The listing builds one solid part. Answer for the finished solid, in the listing's coordinates (mm). Give positions to 0.01 mm unless a question says otherwise; leave off trailing zeros. Write each loop counter-clockwise with the first axis right and the second up, starting at its lowest first coordinate (ties: lowest second). Pieces come first, ordered by that corner, then holes. Notation, with made-up numbers: (54, 23) - (103, 23) arc R26 cw to (103, 50) - close; hole circle Ø6 at (57.25, -10). An arc over 180 degrees is marked (long way). Answer as CSV lines item,"result". Start each with the question number.
(1) Find section A-A (x = 1). Write down the section's boundary in (y, z) (3 decimals).
(2) Find section C-C (x = 4.75). Write down the section's boundary in (y, z) (3 decimals), then the cut area to 3 significant figures.
(3) Each of these flat-tipped pins is pushed along its axis until it touches: pin 1 Ø1.2 at (x, z) = (9, 28.5) entering from -Y; pin 2 Ø0.7 at (y, z) = (7.5, 43.5) entering from -X; pin 3 Ø1.6 at (x, z) = (7.5, 28.5) entering from -Y. Where does it stop, or does it pass through?
(4) Find section B-B (y = 0.75). Write down the section's boundary in (x, z) (3 decimals), then the cut area to 3 significant figures.
(5) Straight lines are drawn through the part: probe 1 along X at (y, z) = (-5.25, 23.5) (3 decimals); probe 2 along X at (y, z) = (2.5, 11.5) (3 decimals); probe 3 along Y at (x, z) = (4.25, 14) (3 decimals). For each, find the intervals that lie inside material, in ascending order.
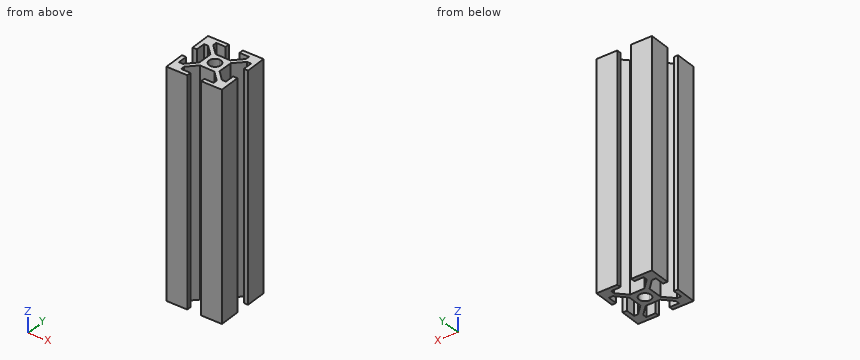
from build123d import *

# Parameters (mm, degrees)
F1_DEPTH = 80
F3_COUNT = 4


with BuildPart() as f1:
    # F0 (on Top) → F1 (new body)
    with BuildSketch(Plane.XY):
        with BuildLine():
            Line((0, 3.655), (-2.594135, 3.655))
            Line((-2.594135, 3.655), (-5.994502, 6.92418))
            Line((-5.994502, 6.92418), (-5.994502, 8.355))
            Line((-5.994502, 8.355), (-2.629502, 8.355))
            Line((-2.629502, 8.355), (-2.629502, 9.855))
            Line((-2.629502, 9.855), (-9.998107, 9.711609))
            Line((-9.998107, 9.711609), (-9.854716, 2.343004))
            Line((-9.854716, 2.343004), (-8.355, 2.372188))
            Line((-8.355, 2.372188), (-8.355, 5.737188))
            Line((-8.355, 5.737188), (-6.92418, 5.737188))
            Line((-6.92418, 5.737188), (-3.655, 2.594135))
            Line((-3.655, 2.594135), (-3.655, 0))
            Line((-3.655, 0), (-2.094884, 0))
            ThreePointArc((-2.094884, 0), (-1.481273, 1.481273), (0, 2.094884))
            Line((0, 2.094884), (0, 3.655))
        make_face()
    extrude(amount=F1_DEPTH)

    # F3: F1 ×4 about axis
    f3_axis = Axis((0, 0, 0.688764), (0, 0, 1))


with BuildPart() as f1_1:
    add(f1.part)
    for i in range(1, F3_COUNT):
        add(f1.part.rotate(f3_axis, i * 360 / F3_COUNT))


solid = f1_1.part
Result set:
1,outline,"(-3.655, 0) - (-1.841, 0) - (-1.841, 80) - (-3.655, 80) - close; (1.841, 0) - (3.655, 0) - (3.655, 80) - (1.841, 80) - close"
2,outline,"(-9.814, 0) - (-8.355, 0) - (-8.355, 80) - (-9.814, 80) - close; (-5.728, 0) - (-3.647, 0) - (-3.647, 80) - (-5.728, 80) - close; (3.733, 0) - (5.897, 0) - (5.897, 80) - (3.733, 80) - close; (8.355, 0) - (9.902, 0) - (9.902, 80) - (8.355, 80) - close"
2,area,"580 mm^2"
3,pin 1,"y = -9.74"
3,pin 2,"x = -9.96"
3,pin 3,"y = -9.78"
4,outline,"(-3.655, 0) - (-1.956, 0) - (-1.956, 80) - (-3.655, 80) - close; (1.956, 0) - (3.655, 0) - (3.655, 80) - (1.956, 80) - close"
4,area,"272 mm^2"
5,probe 1,"-9.804 to -8.355, -6.208 to -4.128, 4.253 to 6.417, 8.355 to 9.911"
5,probe 2,"-9.858 to -8.355, -3.655 to 3.655"
5,probe 3,"-9.823 to -8.355, -5.247 to -3.166, 3.213 to 5.377, 8.355 to 9.892"
